```python
from build123d import *

# Parameters (mm, degrees)
SKETCH1_R           = 63.5
BOSS_EXTRUDE1_DEPTH = 10.16
SKETCH2_R           = 50.8
CUT_EXTRUDE1_DEPTH  = 91.375470123
CIRPATTERN1_COUNT   = 6
CUT_EXTRUDE2_DEPTH  = 90.240886157
SKETCH4_R           = 6.4135
CUT_EXTRUDE3_DEPTH  = 90.240886157
CIRPATTERN2_COUNT   = 6
FILLET1_R           = 1.905
SKETCH5_R           = 31.75
BOSS_EXTRUDE2_DEPTH = 15.24
SKETCH6_R           = 6.4135
CUT_EXTRUDE4_DEPTH  = 90.960923529
FILLET2_R           = 2.54
FILLET3_R           = 5.08
FILLET4_R           = 1.27


with BuildPart() as part:
    # Sketch1 → Boss-Extrude1 (new body)
    with BuildSketch(Plane(origin=(0, 0, 0), x_dir=(1, 0, 0), z_dir=(0, 1, 0))):
        with Locations(Location((0, 0, 0), (0, 0, 270))):
            Circle(SKETCH1_R)
    extrude(amount=BOSS_EXTRUDE1_DEPTH)

    # Sketch2 → Cut-Extrude1 (cut, through all)
    with BuildSketch(Plane(origin=(0, 10.16, 0), x_dir=(1, 0, 0), z_dir=(0, 1, 0))):
        with Locations((-71.842048969, 71.842048969)):
            Circle(SKETCH2_R)
    cut_extrude1 = extrude(amount=-CUT_EXTRUDE1_DEPTH, mode=Mode.SUBTRACT)

    # CirPattern1: Cut-Extrude1 ×6 about axis
    cirpattern1_axis = Axis((0, 0, 0), (0, 1, 0))
    for i in range(1, CIRPATTERN1_COUNT):
        add(cut_extrude1.rotate(cirpattern1_axis, i * 360 / CIRPATTERN1_COUNT), mode=Mode.SUBTRACT)

    # Sketch3 → Cut-Extrude2 (cut, through all)
    with BuildSketch(Plane(origin=(0, 10.16, 0), x_dir=(1, 0, 0), z_dir=(0, 1, 0))):
        with BuildLine():
            Line((-60.481669482, 19.624496442), (-32.880338996, 12.228742229))
            ThreePointArc((-32.880338996, 12.228742229), (-30.545472405, 8.184634663), (-34.58957997, 5.849768072))
            Line((-34.58957997, 5.849768072), (-62.190910456, 13.245522286))
            ThreePointArc((-62.190910456, 13.245522286), (-64.525777048, 17.289629851), (-60.481669482, 19.624496442))
        make_face()
    cut_extrude2 = extrude(amount=-CUT_EXTRUDE2_DEPTH, mode=Mode.SUBTRACT)

    # Sketch4 → Cut-Extrude3 (cut, through all)
    with BuildSketch(Plane(origin=(0, 10.16, 0), x_dir=(1, 0, 0), z_dir=(0, 1, 0))):
        with Locations(Location((0, 0, 0), (0, 0, 270))):
            Circle(SKETCH4_R)
    extrude(amount=-CUT_EXTRUDE3_DEPTH, mode=Mode.SUBTRACT)

    # CirPattern2: Cut-Extrude2 ×6 about axis
    cirpattern2_axis = Axis((0, 0, 0), (0, 1, 0))
    for i in range(1, CIRPATTERN2_COUNT):
        add(cut_extrude2.rotate(cirpattern2_axis, i * 360 / CIRPATTERN2_COUNT), mode=Mode.SUBTRACT)

    # Fillet1
    fillet1_edges = [part.edges().sort_by_distance(p)[0] for p in [
        (-47.175399572, 5.08, 42.505666389),
        (-42.505666389, 5.08, 47.175399572),
        (13.223287112, 5.08, 62.107927658),
        (19.602261269, 5.08, 60.398686684),
        (60.398686684, 5.08, 19.602261269),
        (62.107927658, 5.08, 13.223287112),
        (47.175399572, 5.08, -42.505666389),
        (42.505666389, 5.08, -47.175399572),
        (-13.223287112, 5.08, -62.107927658),
        (-19.602261269, 5.08, -60.398686684),
        (-60.398686684, 5.08, -19.602261269),
        (-62.107927658, 5.08, -13.223287112),
    ]]
    fillet(fillet1_edges, radius=FILLET1_R)

    # Sketch5 → Boss-Extrude2 (add)
    with BuildSketch(Plane(origin=(0, 0, 0), x_dir=(-1, 0, 0), z_dir=(0, -1, 0))):
        with Locations(Location((0, 0, 0), (0, 0, 256.560575533))):
            Circle(SKETCH5_R)
    extrude(amount=BOSS_EXTRUDE2_DEPTH)

    # Sketch6 → Cut-Extrude4 (cut, through all)
    with BuildSketch(Plane(origin=(0, 0, 0), x_dir=(1, 0, 0), z_dir=(0, 1, 0))):
        with Locations(Location((0, 0, 0), (0, 0, 270))):
            Circle(SKETCH6_R)
    extrude(amount=-CUT_EXTRUDE4_DEPTH, mode=Mode.SUBTRACT)

    # Fillet2
    # the kernel refuses this fillet: 2.54 mm, written as the material it adds along each edge
    with BuildSketch(Plane(origin=(0, 0, 0), x_dir=(0.5749992742751929, 0, -0.8181539186381751), z_dir=(-0.8181539186381751, 0, -0.5749992742751929))) as fillet2_piece_1_section:
        with BuildLine():
            CenterArc((31.75 + FILLET2_R, FILLET2_R), FILLET2_R, 180, 90)
            Line((31.75 + FILLET2_R, 0), (31.75, 0))
            Line((31.75, 0), (31.75, FILLET2_R))
        make_face()
    fillet2_piece_1 = revolve(axis=Axis((0, 0, 0), (0, -1, 0)), revolution_arc=79.800837255, mode=Mode.PRIVATE)
    fillet2_piece_1 = fillet2_piece_1 - Plane(origin=(33.734959483, -0.606371024, 9.03925515), x_dir=(-0.2588190451025229, 0, 0.9659258262890678), z_dir=(0, 1, 0)) * Cylinder(3.302, 138, mode=Mode.PRIVATE)
    fillet2_piece_1 = fillet2_piece_1 - Plane(origin=(24.695704333, -0.606371024, -24.695704333), x_dir=(0.7071067811865457, 0, 0.7071067811865495), z_dir=(0, 1, 0)) * Cylinder(3.302, 138, mode=Mode.PRIVATE)
    add(fillet2_piece_1)
    with BuildSketch(Plane(origin=(0, 0, 0), x_dir=(0.9960417148840375, 0, 0.08888701936090508), z_dir=(0.08888701936090508, 0, -0.9960417148840375))) as fillet2_piece_2_section:
        with BuildLine():
            CenterArc((31.75 + FILLET2_R, FILLET2_R), FILLET2_R, 180, 90)
            Line((31.75 + FILLET2_R, 0), (31.75, 0))
            Line((31.75, 0), (31.75, FILLET2_R))
        make_face()
    fillet2_piece_2 = revolve(axis=Axis((0, 0, 0), (0, -1, 0)), revolution_arc=79.800837255, mode=Mode.PRIVATE)
    fillet2_piece_2 = fillet2_piece_2 - Plane(origin=(9.03925515, -0.606371024, 33.734959483), x_dir=(-0.965925826289069, 0, 0.2588190451025186), z_dir=(0, 1, 0)) * Cylinder(3.302, 138, mode=Mode.PRIVATE)
    fillet2_piece_2 = fillet2_piece_2 - Plane(origin=(33.734959483, -0.606371024, 9.03925515), x_dir=(-0.2588190451025229, 0, 0.9659258262890678), z_dir=(0, 1, 0)) * Cylinder(3.302, 138, mode=Mode.PRIVATE)
    add(fillet2_piece_2)
    with BuildSketch(Plane(origin=(0, 0, 0), x_dir=(0.4210424406137115, 0, 0.9070409379967639), z_dir=(0.9070409379967639, 0, -0.4210424406137115))) as fillet2_piece_3_section:
        with BuildLine():
            CenterArc((31.75 + FILLET2_R, FILLET2_R), FILLET2_R, 180, 90)
            Line((31.75 + FILLET2_R, 0), (31.75, 0))
            Line((31.75, 0), (31.75, FILLET2_R))
        make_face()
    fillet2_piece_3 = revolve(axis=Axis((0, 0, 0), (0, -1, 0)), revolution_arc=79.800837255, mode=Mode.PRIVATE)
    fillet2_piece_3 = fillet2_piece_3 - Plane(origin=(9.03925515, -0.606371024, 33.734959483), x_dir=(-0.965925826289069, 0, 0.2588190451025186), z_dir=(0, 1, 0)) * Cylinder(3.302, 138, mode=Mode.PRIVATE)
    fillet2_piece_3 = fillet2_piece_3 - Plane(origin=(-24.695704333, -0.606371024, 24.695704333), x_dir=(-0.7071067811865459, 0, -0.7071067811865491), z_dir=(0, 1, 0)) * Cylinder(3.302, 138, mode=Mode.PRIVATE)
    add(fillet2_piece_3)
    with BuildSketch(Plane(origin=(0, 0, 0), x_dir=(-0.5749992742751904, 0, 0.8181539186381769), z_dir=(0.8181539186381769, 0, 0.5749992742751904))) as fillet2_piece_4_section:
        with BuildLine():
            CenterArc((31.75 + FILLET2_R, FILLET2_R), FILLET2_R, 180, 90)
            Line((31.75 + FILLET2_R, 0), (31.75, 0))
            Line((31.75, 0), (31.75, FILLET2_R))
        make_face()
    fillet2_piece_4 = revolve(axis=Axis((0, 0, 0), (0, -1, 0)), revolution_arc=79.800837255, mode=Mode.PRIVATE)
    fillet2_piece_4 = fillet2_piece_4 - Plane(origin=(-24.695704333, -0.606371024, 24.695704333), x_dir=(-0.7071067811865459, 0, -0.7071067811865491), z_dir=(0, 1, 0)) * Cylinder(3.302, 138, mode=Mode.PRIVATE)
    fillet2_piece_4 = fillet2_piece_4 - Plane(origin=(-33.734959483, -0.606371024, -9.03925515), x_dir=(0.2588190451025228, 0, -0.9659258262890678), z_dir=(0, 1, 0)) * Cylinder(3.302, 138, mode=Mode.PRIVATE)
    add(fillet2_piece_4)
    with BuildSketch(Plane(origin=(0, 0, 0), x_dir=(-0.9960417148840376, 0, -0.08888701936090405), z_dir=(-0.08888701936090405, 0, 0.9960417148840376))) as fillet2_piece_5_section:
        with BuildLine():
            CenterArc((31.75 + FILLET2_R, FILLET2_R), FILLET2_R, 180, 90)
            Line((31.75 + FILLET2_R, 0), (31.75, 0))
            Line((31.75, 0), (31.75, FILLET2_R))
        make_face()
    fillet2_piece_5 = revolve(axis=Axis((0, 0, 0), (0, -1, 0)), revolution_arc=79.800837255, mode=Mode.PRIVATE)
    fillet2_piece_5 = fillet2_piece_5 - Plane(origin=(-33.734959483, -0.606371024, -9.03925515), x_dir=(0.2588190451025228, 0, -0.9659258262890678), z_dir=(0, 1, 0)) * Cylinder(3.302, 138, mode=Mode.PRIVATE)
    fillet2_piece_5 = fillet2_piece_5 - Plane(origin=(-9.03925515, -0.606371024, -33.734959483), x_dir=(0.9659258262890689, 0, -0.25881904510251885), z_dir=(0, 1, 0)) * Cylinder(3.302, 138, mode=Mode.PRIVATE)
    add(fillet2_piece_5)
    with BuildSketch(Plane(origin=(0, 0, 0), x_dir=(-0.4210424406088149, 0, -0.907040937999037), z_dir=(-0.907040937999037, 0, 0.4210424406088149))) as fillet2_piece_6_section:
        with BuildLine():
            CenterArc((31.75 + FILLET2_R, FILLET2_R), FILLET2_R, 180, 90)
            Line((31.75 + FILLET2_R, 0), (31.75, 0))
            Line((31.75, 0), (31.75, FILLET2_R))
        make_face()
    fillet2_piece_6 = revolve(axis=Axis((0, 0, 0), (0, -1, 0)), revolution_arc=79.800837255, mode=Mode.PRIVATE)
    fillet2_piece_6 = fillet2_piece_6 - Plane(origin=(24.695704333, -0.606371024, -24.695704333), x_dir=(0.7071067811865457, 0, 0.7071067811865495), z_dir=(0, 1, 0)) * Cylinder(3.302, 138, mode=Mode.PRIVATE)
    fillet2_piece_6 = fillet2_piece_6 - Plane(origin=(-9.03925515, -0.606371024, -33.734959483), x_dir=(0.9659258262890689, 0, -0.25881904510251885), z_dir=(0, 1, 0)) * Cylinder(3.302, 138, mode=Mode.PRIVATE)
    add(fillet2_piece_6)

    # Fillet3
    fillet3_edges = [part.edges().sort_by_distance(p)[0] for p in [
        (0, -15.24, -6.4135),
    ]]
    fillet(fillet3_edges, radius=FILLET3_R)

    # Fillet4
    fillet4_edges = [part.edges().sort_by_distance(p)[0] for p in [
        (0, 10.16, -6.4135),
    ]]
    fillet(fillet4_edges, radius=FILLET4_R)


solid = part.part
```
Input: part model. Units: mm. Frame: model coordinates. A direction names the side the tool comes from. Coordinates: 2 decimals unless noted, no trailing zeros. Write each loop counter-clockwise with the first axis right and the second up, starting at its lowest first coordinate (ties: lowest second). Pieces come first, ordered by that corner, then holes. Notation, with made-up numbers: (1.5, -23.5) -> (24.5, -23.5) arc R32 ccw to (24.5, 6.5) -> close; hole circle Ø7 at (-35.75, -24.75). An arc over 180 degrees is marked (long way). Write each question's results on one line, items separated by ' | '.
Item 1: Material intervals for probe 1 along Z at (x, y) = (-35, 2.75); probe 2 along X at (y, z) = (-2.75, 0); probe 3 along X at (y, z) = (-2.25, 0), sorted ascending.
Conclusion:
probe 1: z = -36.87 to -12.8, -5.96 to 30.33, 39.67 to 48.09 | probe 2: x = -31.75 to -6.41, 6.41 to 31.75 | probe 3: x = -31.77 to -6.41, 6.41 to 31.77
Item 2: Mould query, pull axis X, two halves, no side actions, for faces 4 (the flat face through (13, -15.24, -4)), 5 (the flat face through (31.58, 5.15, -36.25)), 6 (the cylindrical face through (36.192, 5.151, 35.652)), 7 (the cylindrical face through (47.14, 5.01, -41.62)). Classes: +X half, -X half, draft (parallel to the pull), parting line (faces both ways), or undercut.
Conclusion:
face 4: draft | face 5: undercut | face 6: +X half | face 7: undercut
Item 3: Section query B-B on x = 0. Return loops of the section in (y, z), plus the area to 3 significant figures.
Conclusion:
outline: (-15.24, -31.75) -> (-2.54, -31.75) arc R2.54 cw to (0, -34.29) -> (0, -54.67) -> (10.16, -54.67) -> (10.16, -7.68) arc R1.27 ccw to (8.89, -6.41) -> (-10.16, -6.41) arc R5.08 ccw to (-15.24, -11.49) -> close; (-15.24, 11.49) arc R5.08 ccw to (-10.16, 6.41) -> (8.89, 6.41) arc R1.27 ccw to (10.16, 7.68) -> (10.16, 54.67) -> (0, 54.67) -> (0, 34.29) arc R2.54 cw to (-2.54, 31.75) -> (-15.24, 31.75) -> close | area: 1,740 mm^2
Item 4: Pin query (flat end, axial travel): pin 1 Ø0.5 at (x, z) = (8.5, 30.5) entering from +Y; pin 2 Ø24 at (x, z) = (-26, -47.5) entering from -Y; pin 3 Ø5 at (x, y) = (30, 7) entering from -Z. Return the tip coordinate at first contact, or that it passes through.
Conclusion:
pin 1: stops at y = 10.16 | pin 2: stops at y = 0 | pin 3: stops at z = -47.72
Item 5: Set-up query: faces 1 (the flat face through (9.32, 5.15, 47.54)), 2 (the cylindrical face through (12.78, 5.15, -49.17)), 3 (the flat face through (-30, 0, -31)). Return all of +Z, -Z, +X, -X, +Y, -Y with unobstructed straight access to the full face (end or side cutting, diameter ignored); none if empty.
Conclusion:
face 1: +Y, -Y | face 2: -Z, +Y, -Y | face 3: -Z, -X, -Y
Item 6: Section query D-D on z = 44. Return loops of the section in (x, y).
Conclusion:
outline: (-39.33, 0) -> (8.37, 0) -> (8.37, 10.16) -> (-39.33, 10.16) -> close; (15.21, 0) -> (29.35, 0) -> (29.35, 10.16) -> (15.21, 10.16) -> close
Item 7: Section query A-A on z = 0. Return loops of the section in (x, y), plus the area to 3 significant figures.
Conclusion:
outline: (-54.67, 0) -> (-34.29, 0) arc R2.54 cw to (-31.75, -2.54) -> (-31.75, -15.24) -> (-11.49, -15.24) arc R5.08 ccw to (-6.41, -10.16) -> (-6.41, 8.89) arc R1.27 ccw to (-7.68, 10.16) -> (-54.67, 10.16) -> close; (6.41, -10.16) arc R5.08 ccw to (11.49, -15.24) -> (31.75, -15.24) -> (31.75, -2.54) arc R2.54 cw to (34.29, 0) -> (54.67, 0) -> (54.67, 10.16) -> (7.68, 10.16) arc R1.27 ccw to (6.41, 8.89) -> close | area: 1,740 mm^2
Item 8: Section query C-C on y = -4. Return loops of the section in (x, z), plus the area to 3 significant figures.
Conclusion:
outline: circle Ø63.5 at (0, 0); hole circle Ø12.83 at (0, 0) | area: 3,040 mm^2
